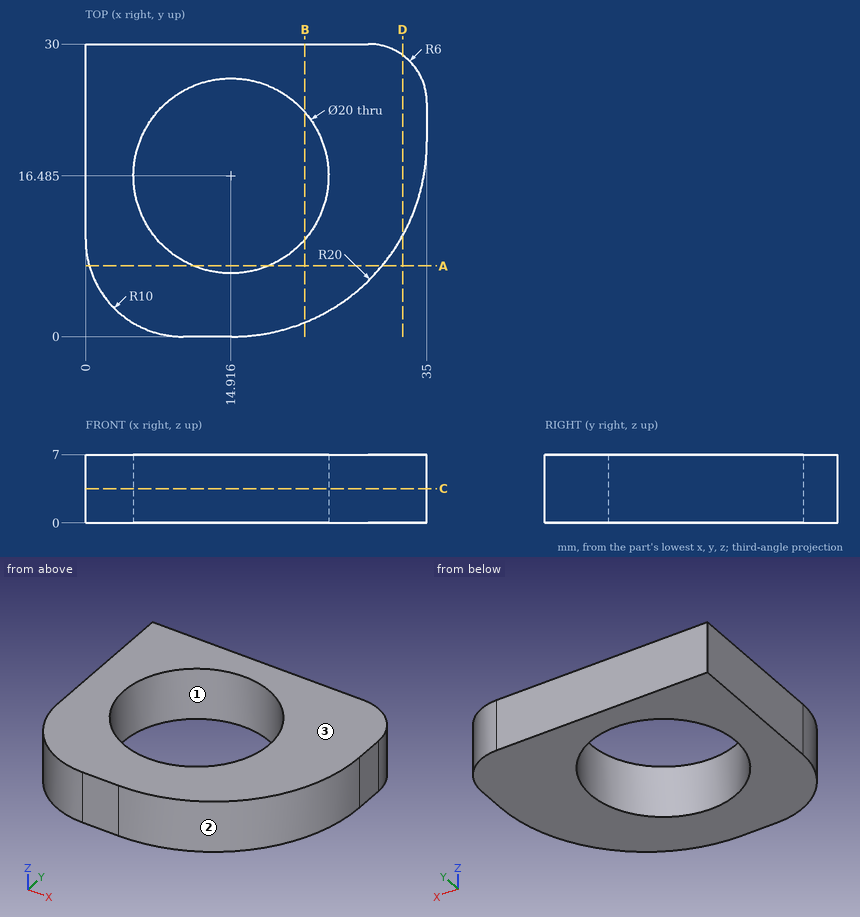
Source: three-view drawing plus pictorial views. Frame: mm from the lowest corner of the part. Give positions to 0.01 mm unless a question says otherwise; leave off trailing zeros. Write each loop counter-clockwise with the first axis right and the second up, starting at its lowest first coordinate (ties: lowest second). Pieces come first, ordered by that corner, then holes. Notation, with made-up numbers: (0.5, -36.75) - (17.5, -36.75) arc R20 ccw to (17.5, -25.75) - close; hole circle Ø7 at (78.25, -18). An arc over 180 degrees is marked (long way). Write item = value, one per line. Start each with the question number.
1. Section query C-C, the plane z = 3.5. Output: boundary loops of the cut face in (x, y) (1 decimal).
2. First-contact query: pin 1 Ø1.5 at (x, z) = (31, 4.5) entering from -Y. Flat tip, straight axial feed; report the tip coordinate or a pass-through.
3. Section query D-D, the plane x = 32.5. Output: boundary loops of the cut face in (y, z), then the cut area to 3 significant figures.
4. Section query A-A, the plane y = 7.25. Output: boundary loops of the cut face in (x, z) (1 decimal).
5. Section query B-B, the plane x = 22.5. Output: boundary loops of the cut face in (y, z).
6. Mould query, pull axis X, two halves, no side actions, for the marked faces 1, 2 and 3. Classes: released by +X, released by -X, zero draft, split by the parting line, or undercut.
7. Ray query, L1, parallel to X at y = 18.75, z = 3 (1 decimal); L2, parallel to X at y = 21, z = 4.5; L3, parallel to Y at x = 10.5, z = 3. Return the intervals inside material, ascending.
Check sheet entries:
q1.outline = (0, 10) arc R10 ccw to (10, 0) - (15, 0) arc R20 ccw to (35, 20) - (35, 24) arc R6 ccw to (29, 30) - (0, 30) - close; hole circle Ø20 at (14.9, 16.5)
q2.pin_1 = 7.06
q3.outline = (10.32, 0) - (28.87, 0) - (28.87, 7) - (10.32, 7) - close
q3.area = 130 mm2
q4.outline = (0.4, 0) - (11.1, 0) - (11.1, 7) - (0.4, 7) - close; (18.8, 0) - (30.4, 0) - (30.4, 7) - (18.8, 7) - close
q5.outline = (1.46, 0) - (9.97, 0) - (9.97, 7) - (1.46, 7) - close; (23, 0) - (30, 0) - (30, 7) - (23, 7) - close
q6.face_1 = undercut
q6.face_2 = released by +X
q6.face_3 = zero draft
q7.L1 = 0 to 5.2, 24.7 to 35
q7.L2 = 0 to 5.99, 23.84 to 35
q7.L3 = 0 to 7.51, 25.46 to 30
